Geometry check sheet. Reference: the model listing, model coordinates, mm. Give positions to 0.01 mm unless a question says otherwise; leave off trailing zeros. Write each loop counter-clockwise with the first axis right and the second up, starting at its lowest first coordinate (ties: lowest second). Pieces come first, ordered by that corner, then holes.
(1) Thickness scan on line 1 along Y through (x, z) = (130, 0.5); line 2 along Y through (x, z) = (10, 3.25); line 3 along X through (y, z) = (18, 2.6). Record the ranges inside material, lowest first.
(2) Cross-section at B-B (y = 9). Record the boundary of the cut face in (x, z), and give its area (3 significant figures).
(3) Cross-section at A-A (z = 2.6). Record the boundary of the cut face in (x, y).
(4) Depth check by flat-ended pin: P1, Ø2.5, axis at x = 10, y = 15, coming from the -Z side; P2, Ø5.5, axis at x = 129.5, y = 29.5, coming from the +Z side. Enter the tip coordinate at first touch or a pass-through.
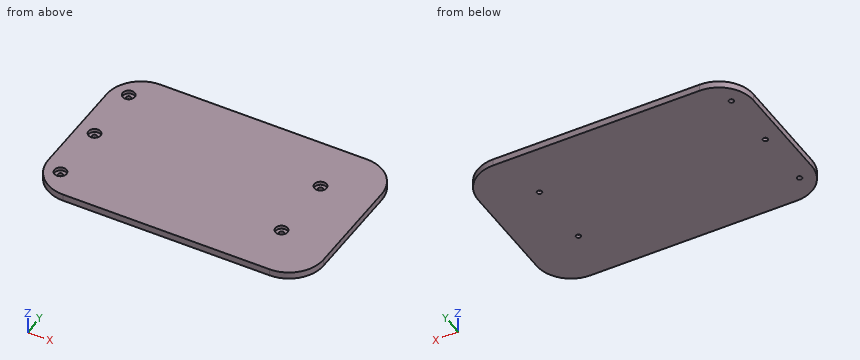
```python
from build123d import *

# Parameters (mm, degrees)
SKETCH1_W           = 160
SKETCH1_H           = 100
BOSS_EXTRUDE1_DEPTH = 4
FILLET1_R           = 20
SKETCH2_R           = 1.4
CUT_EXTRUDE1_DEPTH  = 4
SKETCH3_R           = 3.5
CUT_EXTRUDE2_DEPTH  = 2


with BuildPart() as part:
    # Sketch1 → Boss-Extrude1 (new body)
    with BuildSketch(Plane.XY):
        with Locations((80, 50)):
            Rectangle(SKETCH1_W, SKETCH1_H)
    extrude(amount=BOSS_EXTRUDE1_DEPTH)

    # Fillet1
    fillet1_edges = [part.edges().sort_by_distance(p)[0] for p in [
        (0, 100, 2),
        (160, 100, 2),
        (160, 0, 2),
        (0, 0, 2),
    ]]
    fillet(fillet1_edges, radius=FILLET1_R)

    # Sketch2 → Cut-Extrude1 (cut)
    with BuildSketch(Plane.XY.offset(4)):
        with Locations((130, 30)):
            Circle(SKETCH2_R)
        with Locations((130, 70)):
            Circle(SKETCH2_R)
        with Locations((10, 15)):
            Circle(SKETCH2_R)
        with Locations((10, 50)):
            Circle(SKETCH2_R)
        with Locations((10, 85)):
            Circle(SKETCH2_R)
    extrude(amount=-CUT_EXTRUDE1_DEPTH, mode=Mode.SUBTRACT)

    # Sketch3 → Cut-Extrude2 (cut)
    with BuildSketch(Plane.XY.offset(4)):
        with Locations((130, 30)):
            Circle(SKETCH3_R)
        with Locations((130, 70)):
            Circle(SKETCH3_R)
        with Locations((10, 85)):
            Circle(SKETCH3_R)
        with Locations((10, 50)):
            Circle(SKETCH3_R)
        with Locations((10, 15)):
            Circle(SKETCH3_R)
    extrude(amount=-CUT_EXTRUDE2_DEPTH, mode=Mode.SUBTRACT)


solid = part.part
```
Reply:
1. line 1: y = 0 to 28.6, 31.4 to 68.6, 71.4 to 100
1. line 2: y = 2.68 to 11.5, 18.5 to 46.5, 53.5 to 81.5, 88.5 to 97.32
1. line 3: x = 0.1 to 8.2, 11.8 to 159.9
2. outline: (3.3, 0) - (156.7, 0) - (156.7, 4) - (3.3, 4) - close
2. area: 614 mm2
3. outline: (0, 20) arc R20 ccw to (20, 0) - (140, 0) arc R20 ccw to (160, 20) - (160, 80) arc R20 ccw to (140, 100) - (20, 100) arc R20 ccw to (0, 80) - close; hole circle Ø7 at (10, 15); hole circle Ø7 at (10, 50); hole circle Ø7 at (10, 85); hole circle Ø7 at (130, 30); hole circle Ø7 at (130, 70)
4. P1: passes through
4. P2: stops at z = 2
